The listing builds one solid part. Answer for the finished solid, in the listing's coordinates (mm). A direction names the side the tool comes from. Coordinates: 2 decimals unless noted, no trailing zeros. Write each loop counter-clockwise with the first axis right and the second up, starting at its lowest first coordinate (ties: lowest second). Pieces come first, ordered by that corner, then holes. Notation, with made-up numbers: M -2,58 L 13,58 A8 ccw 13,69 Z; hole C -29.5,33 d3. An arc over 180 degrees is marked long. Answer as a JSON object with one key per item and string values. Group by question number.
from build123d import *

# Parameters (mm, degrees)
SKETCH_1_W             = 43
SKETCH_1_H             = 60
EXTRUDE_3_DEPTH        = 16
SKETCH_2_R             = 3
CUT_EXTRUDE_1_DEPTH    = 76.531450403
HOLE_WIZARD_M6_1_D     = 5
HOLE_WIZARD_M6_1_DEPTH = 10
HOLE_WIZARD_M6_1_TIP   = 1.502151548


with BuildPart() as part:
    # 草图1 → 凸台-拉伸3 (new body)
    with BuildSketch(Plane.XY):
        with Locations((-21.5, 30)):
            Rectangle(SKETCH_1_W, SKETCH_1_H)
    extrude(amount=EXTRUDE_3_DEPTH)

    # 草图2 → 切除-拉伸1 (cut, through all)
    with BuildSketch(Plane(origin=(0, 0, 0), x_dir=(-1, 0, 0), z_dir=(0, 0, -1))):
        with Locations((15, 52)):
            Circle(SKETCH_2_R)
        with Locations((15, 6)):
            Circle(SKETCH_2_R)
    extrude(amount=-CUT_EXTRUDE_1_DEPTH, mode=Mode.SUBTRACT)

    # M6 螺纹孔1
    with Locations(Plane.ZY.offset(43)):
        with Locations((8, 42), (8, 18)):
            Hole(HOLE_WIZARD_M6_1_D / 2, depth=HOLE_WIZARD_M6_1_DEPTH)
            with Locations((0, 0, -(HOLE_WIZARD_M6_1_DEPTH + HOLE_WIZARD_M6_1_TIP / 2))):  # 118° drill point
                Cone(0, HOLE_WIZARD_M6_1_D / 2, HOLE_WIZARD_M6_1_TIP, mode=Mode.SUBTRACT)


solid = part.part
Item 1: A tool of negligible diameter and unlimited length cuts with its end or side. For faces 1 (the face through (-37.93, 20.48, 8.33)), 2 (the face through (-12.6, 4.2, 7.9)), from which of +Z, -Z, +X, -X, +Y, -Y can it reach the whole face along a straight path? Write none if from no direction.
Item 2: Consider L1, parallel to Y at x = -15, z = 9.25; L2, parallel to Y at x = -35.75, z = 8; L3, parallel to Z at x = -36.25, y = 18. Determine where each line is inside the solid, lowest interval first. Write a range as from..to.
Item 3: A cutting plane is placed at C-C, the plane z = 12.75. Write down the section's boundary in (x, y).
Item 4: Flat-ended cylindrical pins translate along their axes: pin 1 Ø10 at (x, y) = (-38, 38) entering from -Z; pin 2 Ø4.5 at (y, z) = (42, 8) entering from -X. Find the tip coordinate at first contact, or state that the pin passes through.
Item 5: A cutting plane is placed at D-D, the plane x = -35. Write down the section's boundary in (y, z).
Item 6: A cutting plane is placed at B-B, the plane x = -15. Write down the section's boundary in (y, z).
Item 7: For a pull along Z with two mould halves and no side action, classify faces 3 (the face through (-37.93, 39.56, 8.54)), 4 (the face through (-15, 55, 8)), 5 (the face through (-22, 30, 0)) as +Z half, -Z half, draft (parallel to the pull), parting line (faces both ways), or undercut.
Item 8: A cutting plane is placed at A-A, the plane y = 52. Write down the section's boundary in (x, z), and give its area (3 significant figures).
Answer:
{
 "1": {"face 1": "-X", "face 2": "+Z, -Z"},
 "2": {"L1": "0..3, 9..49, 55..60", "L2": "0..15.5, 20.5..39.5, 44.5..60", "L3": "0..5.5, 10.5..16"},
 "3": {"outline": "M -43,0 L 0,0 L 0,60 L -43,60 Z; hole C -15,6 d6; hole C -15,52 d6"},
 "4": {"pin 1": "z = 0", "pin 2": "x = -32.85"},
 "5": {"outline": "M 0,0 L 60,0 L 60,16 L 0,16 Z; hole C 18,8 d5; hole C 42,8 d5"},
 "6": {"outline": "M 0,0 L 3,0 L 3,16 L 0,16 Z; M 9,0 L 49,0 L 49,16 L 9,16 Z; M 55,0 L 60,0 L 60,16 L 55,16 Z"},
 "7": {"face 3": "undercut", "face 4": "draft", "face 5": "-Z half"},
 "8": {"outline": "M -43,0 L -18,0 L -18,16 L -43,16 Z; M -12,0 L 0,0 L 0,16 L -12,16 Z", "area": "592 mm2"}
}
